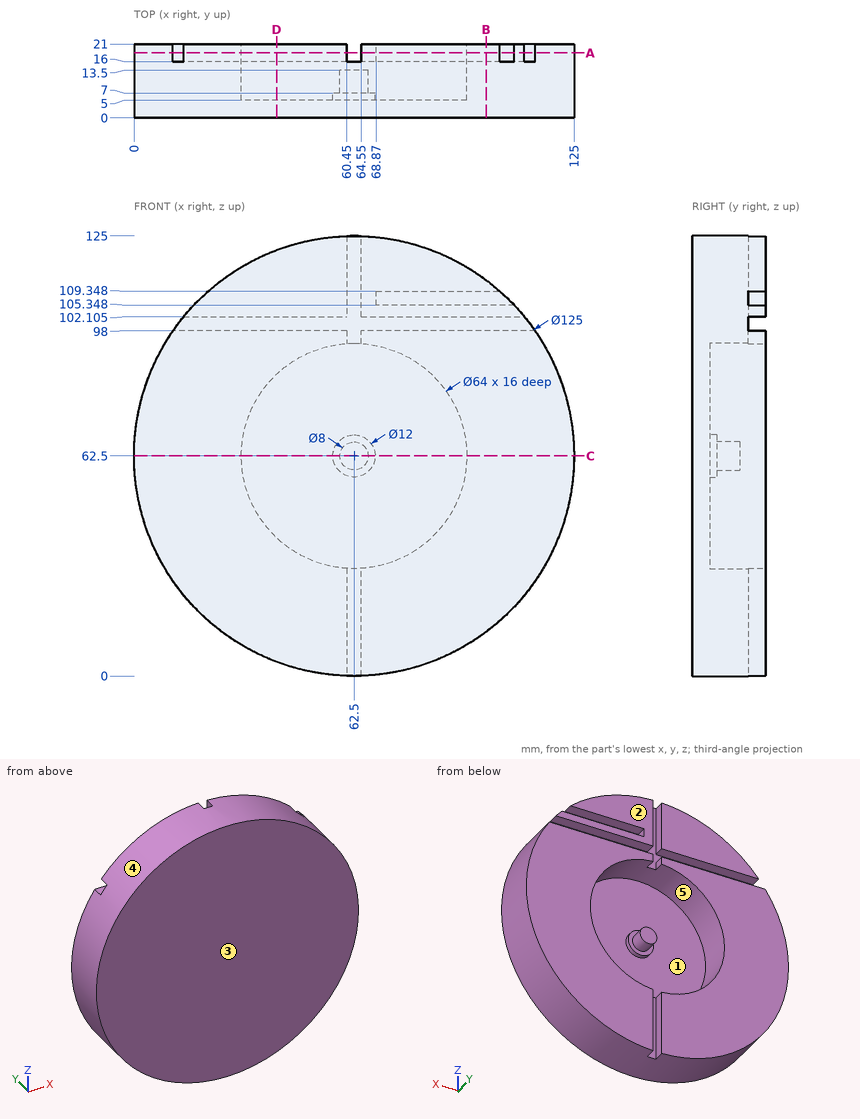
For this review, use the dimensioned drawing (mm, ordinates from the lowest corner) and the shaded views. A direction names the side the tool comes from. Round coordinates to 2 decimals unless told otherwise and drop trailing zeros. Order: outer loops, then holes, each group sorted by start corner. A loop starts at its lowest first (then second) coordinate and runs counter-clockwise, first axis right, second up. Notation, with made-up numbers: M -39.5,22.5 L -0.5,22.5 A13 cw -0.5,47.5 Z; hole C -9.5,65 d9. An arc over 180 degrees is marked long. Write each question's results on one line, items separated by ' | '. Start each with the question number.
1. Clearance check with flat-ended pins moving along their axes: pin 1 Ø2.5 at (y, z) = (17.5, 112.5) entering from +X; pin 2 Ø1.5 at (x, y) = (84, 18.5) entering from +Z (1 decimal); pin 3 Ø3 at (y, z) = (18.5, 108.5) entering from +X; pin 4 Ø3 at (x, z) = (43.5, 64) entering from -Y. State where each tip first meets the part, or that it passes through.
2. Tool access review of the marked faces 1 and 2: name each direction out of +Z, -Z, +X, -X, +Y, -Y from which nothing blocks a thin tool from reaching the whole face with its end or side.
3. Add section D-D (x = 40.5). State the section outline as (y, z) points (1 decimal).
4. Add section A-A (y = 18.5). State how many separate pieces and enclosed holes the cut face has, then the cut area to 3 significant figures.
5. Add section B-B (x = 100). State the section outline as (y, z) points (1 decimal).
6. Add section C-C (z = 62.5). State the section outline as (x, y) points.
7. Draft analysis for pull direction Z (two halves, no side actions). For the marked faces 3, 4 and 5, state which applies: pulls with the +Z half, pulls with the -Z half, needs draft (parallel to the pull), parting line crosses it, or undercut.
8. To check wall thickness, follow L1, parallel to X at y = 9, z = 62.5; L2, parallel to X at y = 17.5, z = 62.5; L3, parallel to Y at x = 68, z = 74. State the ranges of each line that lie inside material, in increasing order. Write a range as [from, to].
Output values:
1) pin 1: x = 101.61 | pin 2: z = 121.5 | pin 3: x = 103.87 | pin 4: y = 0
2) face 1: +Y | face 2: +Z, -Z, +X, -X, +Y
3) outline: M 0,4 L 21,4 L 21,39.3 L 5,39.3 L 5,85.7 L 21,85.7 L 21,98 L 16,98 L 16,102.1 L 21,102.1 L 21,121 L 0,121 Z
4) separate pieces: 4 | enclosed holes: 0 | area: 8,260 mm^2
5) outline: M 0,12.5 L 21,12.5 L 21,98 L 16,98 L 16,102.1 L 21,102.1 L 21,105.3 L 16,105.3 L 16,109.3 L 21,109.3 L 21,112.5 L 0,112.5 Z
6) outline: M 0,0 L 125,0 L 125,21 L 94.5,21 L 94.5,5 L 68.5,5 L 68.5,7 L 66.5,7 L 66.5,13.5 L 58.5,13.5 L 58.5,7 L 56.5,7 L 56.5,5 L 30.5,5 L 30.5,21 L 0,21 Z
7) face 3: needs draft | face 4: parting line crosses it | face 5: undercut
8) L1: [0, 30.5], [58.5, 66.5], [94.5, 125] | L2: [0, 30.5], [94.5, 125] | L3: [0, 5]
